from build123d import *
from build123d.topology import SkipClean

# Parameters (mm, degrees)
BOSS_EXTRUDE1_DEPTH     = 8
BOSS_EXTRUDE2_REACH     = 29.616
SKETCH3_W               = 8
SKETCH3_H               = 20
BOSS_EXTRUDE3_DEPTH     = 6
SKETCH5_R               = 1.5
CUT_EXTRUDE1_DEPTH      = 30
CUT_EXTRUDE2_DEPTH      = 30
CUT_EXTRUDE2_DEPTH_BACK = 2.5
SKETCH6_R               = 1.872244448
SKETCH6_R_2             = 2.25
SKETCH6_R_3             = 2.800873709
SKETCH7_R               = 2.800873709
CUT_EXTRUDE3_DEPTH      = 32.5
BOSS_EXTRUDE4_DEPTH     = 0.45
BOSS_EXTRUDE5_REACH     = 34.303
SKETCH9_W               = 3.185015847
SKETCH9_H               = 14
SKETCH10_W              = 39.020325901
SKETCH10_H              = 14
BOSS_EXTRUDE6_DEPTH     = 0.45
BOSS_EXTRUDE7_DEPTH     = 5
BOSS_EXTRUDE8_REACH     = 71.397
SKETCH12_W              = 4.7
SKETCH12_H              = 62.1
BOSS_EXTRUDE10_REACH    = 73.051
BOSS_EXTRUDE12_REACH    = 73.051
SKETCH15_W              = 0.383636216
SKETCH15_H              = 14
SKETCH16_W              = 44.125949978
SKETCH16_H              = 62.1
BOSS_EXTRUDE13_DEPTH    = 5
FILLET1_R               = 7
SKETCH17_R              = 2.2
CUT_EXTRUDE8_DEPTH      = 20
CUT_EXTRUDE9_DEPTH      = 20
BOSS_EXTRUDE14_DEPTH    = 20
SKETCH20_R              = 1.7
CUT_EXTRUDE10_DEPTH     = 20
SKETCH21_W              = 4
SKETCH21_H              = 10
CUT_EXTRUDE11_DEPTH     = 11


with BuildPart() as part:
    # Sketch1 → Boss-Extrude1 (new body)
    with BuildSketch(Plane.XY):
        Polygon((-9.8, -9.9), (14.667227969, -10), (14.667227969, 10), (-9.8, 10), align=None)
    extrude(amount=BOSS_EXTRUDE1_DEPTH)

    # Boss-Extrude2: up to this plane
    boss_extrude2_end = Plane(origin=(-21.20832686, 0.146710491, 44.5), z_dir=(0.9999916479126735, -0.0040870655604918985, 1.0611945867115664e-14))
    # Sketch3 → Boss-Extrude2 (add, up to the surface)
    with BuildSketch(Plane.ZY.offset(9.8), mode=Mode.PRIVATE) as boss_extrude2_sk1:
        with Locations((4, 0)):
            Rectangle(SKETCH3_W, SKETCH3_H)
    boss_extrude2_tool1 = split(extrude(boss_extrude2_sk1.sketch, amount=BOSS_EXTRUDE2_REACH, mode=Mode.PRIVATE), bisect_by=boss_extrude2_end, keep=Keep.BOTH, mode=Mode.PRIVATE)
    add(boss_extrude2_tool1.solids().sort_by_distance((-9.8, 0, 4))[0])

    # Sketch4 → Boss-Extrude3 (add)
    with BuildSketch(Plane.XY.offset(8)):
        Polygon((14.667227969, 10), (-8.850453012, 10), (-8.850453012, -9.903880893), (14.667227969, -10), align=None)
    extrude(amount=BOSS_EXTRUDE3_DEPTH)

    # Sketch5 → Cut-Extrude1 (cut)
    with BuildSketch(Plane(origin=(0, 0, 0), x_dir=(-1, 0, 0), z_dir=(0, 0, -1))):
        with Locations((9.8, 7)):
            Circle(SKETCH5_R)
        with Locations((16.600765498, 0.199234502)):
            Circle(SKETCH5_R)
        with Locations((2.999234502, 0.199234502)):
            Circle(SKETCH5_R)
        with Locations((9.8, -6.601530997)):
            Circle(SKETCH5_R)
    extrude(amount=-CUT_EXTRUDE1_DEPTH, mode=Mode.SUBTRACT)

    # Sketch6 → Cut-Extrude2 (cut, two sides: drawn at the far end of the back side and taken through both)
    with BuildSketch(Plane.XY.offset(8).offset(-CUT_EXTRUDE2_DEPTH_BACK)):
        with Locations(Location((-9.8, -6.601530997, 0), (0, 0, 300.475535412))):
            Circle(SKETCH6_R)
        with Locations((-2.999234502, 0.199234502)):
            Circle(SKETCH6_R_2)
        with Locations(Location((-16.600765498, 0.199234502, 0), (0, 0, 180))):
            Circle(SKETCH6_R_2)
        with Locations(Location((-9.8, 7, 0), (0, 0, 65.037759798))):
            Circle(SKETCH6_R_2)
        with Locations(Location((-9.8, 0, 0), (0, 0, 289.81706499))):
            Circle(SKETCH6_R_3)
    extrude(amount=CUT_EXTRUDE2_DEPTH + CUT_EXTRUDE2_DEPTH_BACK, mode=Mode.SUBTRACT)

    # Sketch7 → Cut-Extrude3 (cut)
    with SkipClean():  # the faces are left unmerged after this step: merging them gives an invalid solid
        with BuildSketch(Plane.XY.offset(8)):
            with Locations(Location((-9.8, 0, 0), (0, 0, 180))):
                Circle(SKETCH7_R)
        extrude(amount=-CUT_EXTRUDE3_DEPTH, mode=Mode.SUBTRACT)
    add(part.part.scale(1), mode=Mode.REPLACE)  # the faces are merged on a copy

    # Sketch8 → Boss-Extrude4 (add)
    with BuildSketch(Plane(origin=(-0.040625311, -9.939887537, 0), x_dir=(-0.9999916479126736, 0.004087065560474376, 0), z_dir=(-0.004087065560474377, -0.9999916479126737, 0))):
        Polygon((21.208749342, -8), (21.208749342, -14), (-17.811250658, -14), (-17.811250658, 0), (21.208749342, 0), align=None)
    extrude(amount=BOSS_EXTRUDE4_DEPTH)

    # Boss-Extrude5: up to this face of the body (flat: up to its plane)
    boss_extrude5_end = Plane(part.part.faces().sort_by_distance((-1.218931766, 10, 6.308951595))[0])
    # Sketch9 → Boss-Extrude5 (add, up to the picked face)
    with BuildSketch(Plane(origin=(-0.040625311, -9.939887537, 0), x_dir=(0.9999916479126736, -0.004087065560474399, 0), z_dir=(0.0040870655604743995, 0.9999916479126737, 0)), mode=Mode.PRIVATE) as boss_extrude5_sk1:
        with Locations((16.218742735, -7)):
            Rectangle(SKETCH9_W, SKETCH9_H)
    boss_extrude5_tool1 = split(extrude(boss_extrude5_sk1.sketch, amount=BOSS_EXTRUDE5_REACH, mode=Mode.PRIVATE), bisect_by=boss_extrude5_end, keep=Keep.BOTH, mode=Mode.PRIVATE)
    add(boss_extrude5_tool1.solids().sort_by(Axis((16.177982, -10.006175, 7), (0.0040870655604743995, 0.9999916479126737, 0)))[0])

    # Sketch10 → Boss-Extrude6 (add)
    with BuildSketch(Plane(origin=(0, 10, 0), x_dir=(1, 0, 0), z_dir=(0, 1, 0))):
        with Locations((-1.657892534, -7)):
            Rectangle(SKETCH10_W, SKETCH10_H)
    extrude(amount=BOSS_EXTRUDE6_DEPTH)

    # Sketch11 → Boss-Extrude7 (add)
    with BuildSketch(Plane(origin=(0, 10.45, 0), x_dir=(1, 0, 0), z_dir=(0, 1, 0))):
        Polygon((-21.168055484, 0), (17.852270417, 0), (22.852270417, 0), (22.852270417, -55.1), (22.852270417, -62.1), (17.750476753, -62.1), (-21.168055484, -62.1), align=None)
    extrude(amount=BOSS_EXTRUDE7_DEPTH)

    # Boss-Extrude8: up to this plane
    boss_extrude8_end = Plane(origin=(-0.042464491, -10.389883779, 0), z_dir=(0.004087065560474399, 0.9999916479126736, 0))
    # Sketch12 → Boss-Extrude8 (add, up to the surface)
    with BuildSketch(Plane(origin=(0, 10.45, 0), x_dir=(-1, 0, 0), z_dir=(0, -1, 0)), mode=Mode.PRIVATE) as boss_extrude8_sk1:
        with Locations((-20.502270417, -31.05)):
            Rectangle(SKETCH12_W, SKETCH12_H)
    boss_extrude8_tool1 = split(extrude(boss_extrude8_sk1.sketch, amount=BOSS_EXTRUDE8_REACH, mode=Mode.PRIVATE), bisect_by=boss_extrude8_end, keep=Keep.BOTH, mode=Mode.PRIVATE)
    add(boss_extrude8_tool1.solids().sort_by_distance((20.50227, 10.45, 31.05))[0])

    # Boss-Extrude10: up to this plane
    boss_extrude10_end = Plane(origin=(0, 10.45, 0), z_dir=(0, -1, 0))
    # Sketch13 → Boss-Extrude10 (add, up to the surface)
    with BuildSketch(Plane(origin=(-0.042464491, -10.389883779, 0), x_dir=(-0.9999916479126736, 0.004087065560474399, 0), z_dir=(-0.0040870655604743995, -0.9999916479126737, 0)), mode=Mode.PRIVATE) as boss_extrude10_sk1:
        Polygon((8.908749342, -61.4), (8.908749342, -62.1), (-17.791250658, -62.1), (-18.194886874, -62.1), (-18.194886874, -55.657746708), (-17.791250658, -55.657746708), (8.908749342, -55.657746708), align=None)
    boss_extrude10_tool1 = split(extrude(boss_extrude10_sk1.sketch, amount=-BOSS_EXTRUDE10_REACH, mode=Mode.PRIVATE), bisect_by=boss_extrude10_end, keep=Keep.BOTH, mode=Mode.PRIVATE)
    add(boss_extrude10_tool1.solids().sort_by_distance((4.600565, -10.40886, 58.878873))[0])

    # Boss-Extrude12: up to this plane
    boss_extrude12_end = Plane(origin=(0, 10.45, 0), z_dir=(0, -1, 0))
    # Sketch15 → Boss-Extrude12 (add, up to the surface)
    with BuildSketch(Plane(origin=(-0.042464491, -10.389883779, 0), x_dir=(0.9999916479126736, -0.004087065560474399, 0), z_dir=(-0.0040870655604743995, -0.9999916479126737, 0)), mode=Mode.PRIVATE) as boss_extrude12_sk1:
        with Locations((18.003068766, 7)):
            Rectangle(SKETCH15_W, SKETCH15_H)
    boss_extrude12_tool1 = split(extrude(boss_extrude12_sk1.sketch, amount=-BOSS_EXTRUDE12_REACH, mode=Mode.PRIVATE), bisect_by=boss_extrude12_end, keep=Keep.BOTH, mode=Mode.PRIVATE)
    add(boss_extrude12_tool1.solids().sort_by_distance((17.960454, -10.463464, 7))[0])

    # Sketch16 → Boss-Extrude13 (add)
    with BuildSketch(Plane(origin=(-0.042464491, -10.389883779, 0), x_dir=(-0.9999916479126736, 0.004087065560474399, 0), z_dir=(-0.0040870655604743995, -0.9999916479126737, 0))):
        with Locations((-0.83195114, -31.05)):
            Rectangle(SKETCH16_W, SKETCH16_H)
    extrude(amount=BOSS_EXTRUDE13_DEPTH)

    # Fillet1
    # the kernel refuses this fillet: 7 mm, written as the material it takes off along each edge
    with BuildSketch(Plane(origin=(40.352270417, 15.45, 62.1), x_dir=(0, 0, -1), z_dir=(-1, 0, 0))) as fillet1_piece_1:
        with BuildLine():
            CenterArc((FILLET1_R, FILLET1_R), FILLET1_R, 180, 90)
            Line((0, FILLET1_R), (0, 0))
            Line((0, 0), (FILLET1_R, 0))
        make_face()
    extrude(amount=79.020325901, mode=Mode.SUBTRACT)
    with BuildSketch(Plane(origin=(-38.793600183, -15.231545785, 62.1), x_dir=(0.004087065560474399, 0.9999916479126735, 0), z_dir=(0.9999916479126737, -0.0040870655604743995, 0)), Plane(origin=(40.331688928, -15.55493873, 0), x_dir=(0.004087065560474399, 0.9999916479126735, 0), z_dir=(-0.9999916479126737, 0.0040870655604743995, 0))) as fillet1_piece_2:
        with BuildLine():
            CenterArc((FILLET1_R, -FILLET1_R), FILLET1_R, 90, 90)
            Line((0, -FILLET1_R), (0, 0))
            Line((0, 0), (FILLET1_R, 0))
        make_face()
    extrude(amount=79.125949978, mode=Mode.SUBTRACT)
    with BuildSketch(Plane(origin=(-38.668055484, 15.45, 0), x_dir=(0, -1, 0), z_dir=(1, 0, 0))) as fillet1_piece_3:
        with BuildLine():
            CenterArc((FILLET1_R, -FILLET1_R), FILLET1_R, 90, 90)
            Line((0, -FILLET1_R), (0, 0))
            Line((0, 0), (FILLET1_R, 0))
        make_face()
    extrude(amount=79.020325901, mode=Mode.SUBTRACT)

    # Sketch17 → Cut-Extrude8 (cut)
    with BuildSketch(Plane(origin=(-8.908674935, 0.036410643, 0), x_dir=(0, 0, 1), z_dir=(-0.9999916479126737, 0.0040870655604744, -8.326704424266156e-13))):
        with Locations(Location((58.8, -4.889970557, 0), (0, 0, 270))):
            Circle(SKETCH17_R)
        with Locations(Location((58.8, 5.010029443, 0), (0, 0, 270))):
            Circle(SKETCH17_R)
    extrude(amount=-CUT_EXTRUDE8_DEPTH, mode=Mode.SUBTRACT)

    # Sketch18 → Cut-Extrude9 (cut)
    with BuildSketch(Plane.XY.offset(62.1)):
        Polygon((-3.888198616, -4.949888082), (-3.888198616, -8.374149176), (0.111801384, -8.390497575), (0.111801384, -1.449888082), (-3.888198616, -1.449888082), align=None)
        Polygon((-3.888198616, 8.45), (-3.888198616, 5.046398242), (-3.888198616, 1.546398242), (0.111801384, 1.546398242), (0.111801384, 8.45), align=None)
    extrude(amount=-CUT_EXTRUDE9_DEPTH, mode=Mode.SUBTRACT)

    # Sketch19 → Boss-Extrude14 (add)
    with BuildSketch(Plane(origin=(-21.230846526, 0.086772586, 0), x_dir=(0, 0, 1), z_dir=(-0.9999916479126737, 0.0040870655604743995, 0))):
        with BuildLine():
            Line((34.799540996, -15.389970557), (27.692259446, -15.389970557))
            Line((27.692259446, -15.389970557), (20.584977895, -15.389970557))
            Line((20.584977895, -15.389970557), (26.815853016, -16.790117538))
            ThreePointArc((26.815853016, -16.790117538), (27.692259446, -16.887374052), (28.568665876, -16.790117538))
            Line((28.568665876, -16.790117538), (34.799540996, -15.389970557))
        make_face()
        with BuildLine():
            ThreePointArc((26.815853016, 16.790117538), (27.692259446, 16.887374052), (28.568665876, 16.790117538))
            Line((28.568665876, 16.790117538), (34.799540996, 15.389970557))
            Line((34.799540996, 15.389970557), (20.584977895, 15.389970557))
            Line((20.584977895, 15.389970557), (26.815853016, 16.790117538))
        make_face()
    extrude(amount=-BOSS_EXTRUDE14_DEPTH)

    # Sketch20 → Cut-Extrude10 (cut)
    with BuildSketch(Plane(origin=(-21.230846526, 0.086772586, 0), x_dir=(0, 0, 1), z_dir=(-0.9999916479126737, 0.0040870655604743995, 0))):
        with Locations(Location((27.692259446, -12.889970557, 0), (0, 0, 270))):
            Circle(SKETCH20_R)
        with Locations(Location((27.692259446, 12.889970557, 0), (0, 0, 270))):
            Circle(SKETCH20_R)
    extrude(amount=-CUT_EXTRUDE10_DEPTH, mode=Mode.SUBTRACT)

    # Sketch21 → Cut-Extrude11 (cut)
    with BuildSketch(Plane.XY.offset(62.1)):
        with Locations((14.253029049, 0.04825508)):
            Rectangle(SKETCH21_W, SKETCH21_H)
    extrude(amount=-CUT_EXTRUDE11_DEPTH, mode=Mode.SUBTRACT)


solid = part.part
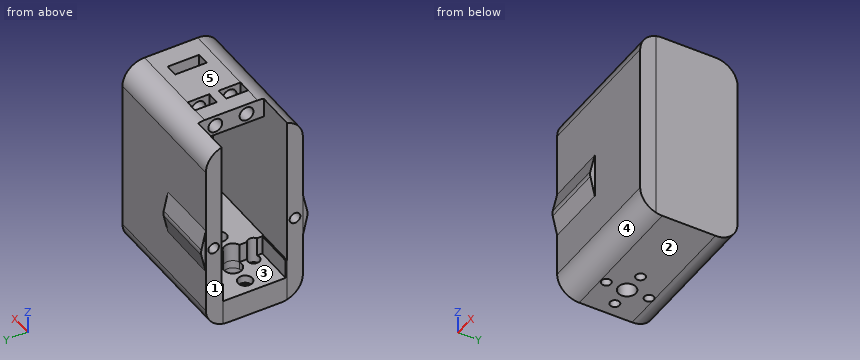
The model under review builds one solid part; all positions refer to its coordinate system, in mm. Face numbers are marked on the shaded views. A direction names the side the tool comes from. Round coordinates to 2 decimals unless told otherwise and drop trailing zeros. Order: outer loops, then holes, each group sorted by start corner. A loop starts at its lowest first (then second) coordinate and runs counter-clockwise, first axis right, second up. Notation, with made-up numbers: (-21, -12) -> (-16, -12) arc R16 ccw to (-16, 19) -> close; hole circle Ø9 at (75, 14.25). An arc over 180 degrees is marked (long way). Return JSON: item names as keys, results as strings.
1. The part is to be moulded in two halves that separate along Y. For the marked faces 3, 4 and 5, say which applies: +Y half, -Y half, draft (parallel to the pull), parting line (faces both ways), or undercut.
Answer block:
{"face 3": "undercut", "face 4": "-Y half", "face 5": "draft"}
2. Insertion check: P1, Ø1.5, axis at y = 12.5, z = 19.5, coming from the -X side; P2, Ø12, axis at x = -5, z = 16, coming from the -Y side; P3, Ø8, axis at x = 9, z = 16, coming from the +Y side; P4, Ø2, axis at x = 16.5, y = 3.5, coming from the -Z side. Each pin has a flat end and moves straight along its axis. Give the tip position at first contact, or say it passes through.
Answer block:
{"P1": "stops at x = -21.17", "P2": "stops at y = -15.69", "P3": "stops at y = 15.45", "P4": "stops at z = 0"}
3. For the marked faces 1 and 2, list the 3-axis set-ups (+Z, -Z, +X, -X, +Y, -Y) from which the entire face can be reached by the end or side of a thin tool; tool diameter is ignored.
Answer block:
{"face 1": "+Z, -Z, -X, +Y", "face 2": "-Z, +X, -X, +Y, -Y"}
4. Take a section at B-B (x = 8.5). State how many separate pieces and enclosed holes the cut face has, then the cut area to 3 significant figures.
Answer block:
{"separate pieces": "1", "enclosed holes": "3", "area": "975 mm²"}
5. For L1, parallel to Z at x = -5.5, y = 8; L2, parallel to X at y = 0, z = 10; L3, parallel to Y at x = 3, z = 57, list the stretches that pass through material, from the lowest coordinate up. Write a range as [from, to].
Answer block:
{"L1": "z = [0, 14], [55.66, 62.1]", "L2": "x = [-7, -5.24], [-0.76, 22.85]", "L3": "y = [-15.14, -6.17], [-3.64, 3.73], [6.26, 15.19]"}
6. Take a section at A-A (z = 18.5). Write out the cut boundary in (x, y), then the cut area to 3 significant figures.
Answer block:
{"outline": "(-21.29, -15.3) -> (22.83, -15.48) -> (22.85, -10.48) -> (22.85, 15.45) -> (-21.17, 15.45) -> (-21.17, 10.45) -> (18.15, 10.45) -> (18.15, -10.46) -> (-21.27, -10.3) -> close", "area": "539 mm²"}
